For this review, take the finished solid that the model builds, in its own axes (mm). Face numbers are marked on the shaded views. A direction names the side the tool comes from. Give positions to 0.01 mm unless a question says otherwise; leave off trailing zeros. Order: outer loops, then holes, each group sorted by start corner. A loop starts at its lowest first (then second) coordinate and runs counter-clockwise, first axis right, second up.
Item 1: Consider section D-D (y = -12). Give the boundary of the cut face in (x, z).
Item 2: The part is to be moulded in two halves that separate along X. For the marked faces 1, 2, 3 and 4, say which applies: released by +X, released by -X, zero draft, split by the parting line, or undercut.
Item 3: For probe 1 along X at (y, z) = (45, 0.7); probe 2 along Y at (x, z) = (32, 1.85); probe 3 along X at (y, z) = (-45, 2.15), list the stretches that pass through material, from the lowest coordinate up.
Item 4: For P1, Ø5, axis at y = 22.5, z = 13, coming from the -X side; P2, Ø3, axis at x = 32, y = 15, coming from the +Z side; P3, Ø5, axis at x = -32, y = -45, coming from the -Z side, all flat-tipped, find the tip position at first contact; note any pin that passes through.
Item 5: Consider section B-B (x = 15.25). Give the boundary of the cut face in (y, z).
Item 6: Consider section A-A (y = 45). Give the boundary of the cut face in (x, z).
Item 7: Machinability: for the marked faces 5, 6, 7, 8 and 9, which of the approach directions +Z, -Z, +X, -X, +Y, -Y give a long, thin tool a straight path to every point of the face, cutting with its end or side? Answer none if there is none.
Item 8: Consider section C-C (x = -32). Give the number of separate pieces and of enclosed holes in the cut face, plus the area to 3 significant figures.
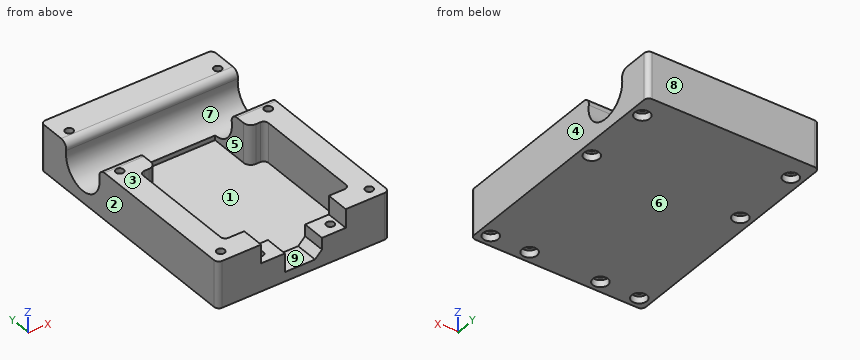
```python
from build123d import *

# Parameters (mm, degrees)
F1_W           = 74
F1_H           = 105
F2_DEPTH       = 3
F3_W           = 74
F3_H           = 105
F4_DEPTH       = 17
F5_R           = 10
F6_DEPTH       = 74.001
F8_D           = 3.4
F8_CBORE_D     = 6.5
F8_CBORE_DEPTH = 3
F9_R           = 2
F10_R          = 3
F11_R          = 2
F12_W          = 36.5
F12_H          = 10
F12_R          = 1.7
F13_DEPTH      = 8
F14_W          = 16
F14_H          = 10
F15_DEPTH      = 16
F16_SIZE       = 3
F17_R          = 3


with BuildPart() as f2:
    # F1 (on face) → F2 (new body)
    with BuildSketch(Plane.XY):
        with Locations((0, 2.5)):
            Rectangle(F1_W, F1_H)
    extrude(amount=F2_DEPTH)

    # F3 (on face) → F4 (join)
    with BuildSketch(Plane.XY.offset(3)):
        with Locations((0, 2.5)):
            Rectangle(F3_W, F3_H)
        Polygon((20, 10), (27, 10), (27, -40), (-27, -40), (-27, 10), (-20, 10), (-20, 30), (20, 30), align=None, mode=Mode.SUBTRACT)
    extrude(amount=F4_DEPTH)

    # F5 (on face) → F6 (cut, through all)
    with BuildSketch(Plane.YZ.offset(37)):
        with Locations((30, 15)):
            Circle(F5_R)
    extrude(amount=-F6_DEPTH, mode=Mode.SUBTRACT)

    # F8 (through all)
    with Locations(Plane(origin=(0, 0, 0), x_dir=(1, 0, 0), z_dir=(0, 0, -1))):
        with Locations((32, -15), (32, -45), (-32, -45), (-32, -15), (32, 45), (-32, 45), (-15.25, 45), (15.25, 45)):
            CounterBoreHole(F8_D / 2, F8_CBORE_D / 2, F8_CBORE_DEPTH)

    # F9
    f9_edges = [f2.edges().sort_by_distance(p)[0] for p in [
        (37, 55, 10),
        (-37, 55, 10),
        (37, -50, 10),
        (-37, -50, 10),
    ]]
    fillet(f9_edges, radius=F9_R)

    # F10
    f10_edges = [f2.edges().sort_by_distance(p)[0] for p in [
        (-20, 10, 11.5),
        (20, 10, 11.5),
    ]]
    fillet(f10_edges, radius=F10_R)

    # F11
    f11_edges = [f2.edges().sort_by_distance(p)[0] for p in [
        (27, 10, 11.5),
        (-27, 10, 11.5),
        (-27, -40, 11.5),
        (27, -40, 11.5),
    ]]
    fillet(f11_edges, radius=F11_R)

    # F12 (on face) → F13 (cut)
    with BuildSketch(Plane.XY.offset(20)):
        with Locations((0, -45)):
            Rectangle(F12_W, F12_H)
        with Locations((-15.25, -45)):
            Circle(F12_R, mode=Mode.SUBTRACT)
        with Locations((15.25, -45)):
            Circle(F12_R, mode=Mode.SUBTRACT)
    extrude(amount=-F13_DEPTH, mode=Mode.SUBTRACT)

    # F14 (on face) → F15 (cut)
    with BuildSketch(Plane.XY.offset(20)):
        with Locations((0, -45)):
            Rectangle(F14_W, F14_H)
    extrude(amount=-F15_DEPTH, mode=Mode.SUBTRACT)

    # F16
    f16_edges = [f2.edges().sort_by_distance(p)[0] for p in [
        (8, -45, 4),
    ]]
    chamfer(f16_edges, length=F16_SIZE)

    # F17
    f17_edges = [f2.edges().sort_by_distance(p)[0] for p in [
        (0, 38.660254, 20),
        (-28.5, 21.339746, 20),
        (28.5, 21.339746, 20),
    ]]
    fillet(f17_edges, radius=F17_R)


solid = f2.part
```
Resolved:
1. outline: (-37, 0) - (37, 0) - (37, 20) - (27, 20) - (27, 3) - (-27, 3) - (-27, 20) - (-37, 20) - close
2. face 1: undercut
2. face 2: released by -X
2. face 3: zero draft
2. face 4: released by +X
3. probe 1: x = -37 to -35.25, -28.75 to 28.75, 35.25 to 37
3. probe 2: y = -50 to -48.25, -41.75 to 11.75, 18.25 to 41.75, 48.25 to 55
3. probe 3: x = -37 to -35.25, -28.75 to -18.5, -12 to 12, 18.5 to 28.75, 35.25 to 37
4. P1: stops at x = -37
4. P2: passes through
4. P3: stops at z = 3
5. outline: (-50, 0) - (-48.25, 0) - (-48.25, 3) - (-46.7, 3) - (-46.7, 12) - (-50, 12) - close; (-43.3, 3) - (-41.75, 3) - (-41.75, 0) - (55, 0) - (55, 20) - (42.85, 20) arc R3 ccw to (39.88, 16.54) arc R10 cw to (30, 5) - (30, 3) - (-40, 3) - (-40, 12) - (-43.3, 12) - close
6. outline: (-37, 0) - (-35.25, 0) - (-35.25, 3) - (-33.7, 3) - (-33.7, 20) - (-37, 20) - close; (-30.3, 3) - (-28.75, 3) - (-28.75, 0) - (28.75, 0) - (28.75, 3) - (30.3, 3) - (30.3, 20) - (-30.3, 20) - close; (33.7, 3) - (35.25, 3) - (35.25, 0) - (37, 0) - (37, 20) - (33.7, 20) - close
7. face 5: +Z
7. face 6: -Z, +X, -X, +Y, -Y
7. face 7: +X, -X
7. face 8: +Z, -Z, +X, -X, +Y
7. face 9: +Z, -Y
8. separate pieces: 4
8. enclosed holes: 0
8. area: 1,610 mm2
